Can you work these out from the model? Positions are in its coordinate system, mm. Face numbers are marked on the shaded views. A direction names the side the tool comes from. Round coordinates to 2 decimals unless told otherwise and drop trailing zeros. Write each loop counter-clockwise with the first axis right and the second up, starting at its lowest first coordinate (ties: lowest second). Pieces come first, ordered by that corner, then holes.
Q1. If we section it at D-D (x = -37): Please give me the cut outline in (y, z).
Q2. If we section it at A-A (x = 2.5): Please give me the cut outline in (y, z).
Q3. If we section it at C-C (y = 36.5): Please give me the cut outline in (x, z), plus the area to 3 significant figures.
Q4. I'm going to push flat-ended pins straight in: pin 1 Ø1.5 at (x, z) = (44.5, 13) entering from -Y; pin 2 Ø1.6 at (x, y) = (47, 51) entering from -Z. Where does each tip first touch, or does it pass through?
Q5. If we section it at B-B (z = 42): Please give me the cut outline in (x, y).
Q6. For the marked faces 1, 2 and 3, which set-ups out of +Z, -Z, +X, -X, +Y, -Y let a thin tool reach every point of the face, with its end or its side?
Q7. We'd pull the mould along X, two halves only. Please class the marked faces 4, 5 and 6: +X half, -X half, draft (parallel to the pull), parting line (faces both ways), or undercut.
Q8. Please list where these lines run through material, in increasing order: line 1 along X through (y, z) = (2.05, 0); line 2 along Y through (x, z) = (4.5, 31.5); line 3 along Z through (x, y) = (-2, 38.5).
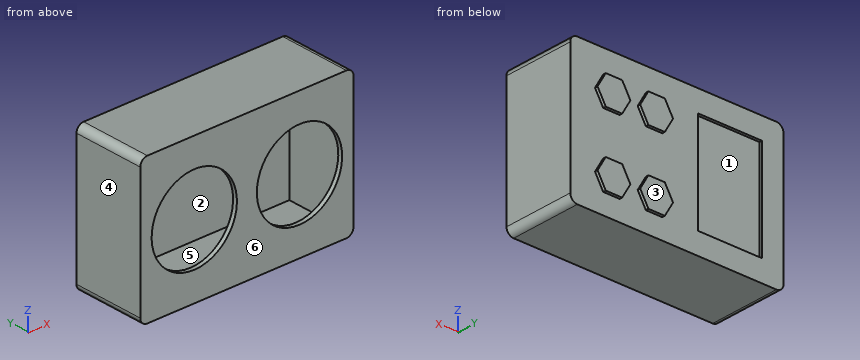
from build123d import *

# Parameters (mm, degrees)
SKETCH1_W           = 150
SKETCH1_H           = 100
BOSS_EXTRUDE1_DEPTH = 50
SHELL1_T            = 3
SKETCH3_R           = 30
CUT_EXTRUDE2_DEPTH  = 5
SKETCH4_W           = 45
SKETCH4_H           = 70
CUT_EXTRUDE3_DEPTH  = 2
BOSS_EXTRUDE2_DEPTH = 2
FILLET1_R           = 5


with BuildPart() as part:
    # Sketch1 → Boss-Extrude1 (new body)
    with BuildSketch(Plane(origin=(0, 0, 0), x_dir=(1, 0, 0), z_dir=(0, 1, 0))):
        Rectangle(SKETCH1_W, SKETCH1_H)
    extrude(amount=BOSS_EXTRUDE1_DEPTH)

    # Shell1 (no face opened: a closed hollow body)
    add(offset(amount=-SHELL1_T, mode=Mode.PRIVATE), mode=Mode.SUBTRACT)

    # Sketch3 → Cut-Extrude2 (cut)
    with BuildSketch(Plane.XZ):
        with Locations(Location((37, 0, 0), (0, 0, 270))):
            Circle(SKETCH3_R)
        with Locations(Location((-37, 0, 0), (0, 0, 270))):
            Circle(SKETCH3_R)
    extrude(amount=-CUT_EXTRUDE2_DEPTH, mode=Mode.SUBTRACT)

    # Sketch4 → Cut-Extrude3 (cut)
    with BuildSketch(Plane(origin=(0, 50, 0), x_dir=(1, 0, 0), z_dir=(0, 1, 0))):
        with Locations((-37.5, 0)):
            Rectangle(SKETCH4_W, SKETCH4_H)
    extrude(amount=-CUT_EXTRUDE3_DEPTH, mode=Mode.SUBTRACT)

    # Sketch5 → Boss-Extrude2 (add)
    with BuildSketch(Plane(origin=(0, 50, 0), x_dir=(1, 0, 0), z_dir=(0, 1, 0))):
        Polygon((57.58863582, -24), (51.815133128, -14), (40.268127744, -14), (34.494625052, -24), (40.268127744, -34), (51.815133128, -34), align=None)
        Polygon((27.58863582, -24), (21.815133128, -14), (10.268127744, -14), (4.494625052, -24), (10.268127744, -34), (21.815133128, -34), align=None)
        Polygon((57.58863582, 26), (51.815133128, 36), (40.268127744, 36), (34.494625052, 26), (40.268127744, 16), (51.815133128, 16), align=None)
        Polygon((27.58863582, 26), (21.815133128, 36), (10.268127744, 36), (4.494625052, 26), (10.268127744, 16), (21.815133128, 16), align=None)
    extrude(amount=BOSS_EXTRUDE2_DEPTH)

    # Fillet1
    fillet1_edges = [part.edges().sort_by_distance(p)[0] for p in [
        (75, 25, 50),
        (-75, 25, 50),
        (-75, 25, -50),
        (75, 25, -50),
    ]]
    fillet(fillet1_edges, radius=FILLET1_R)


solid = part.part
A:
1. outline: (0, -50) - (50, -50) - (50, -35) - (48, -35) - (48, 35) - (50, 35) - (50, 50) - (0, 50) - (0, 30) - (3, 30) - (3, 47) - (47, 47) - (47, -47) - (3, -47) - (3, -30) - (0, -30) - close
2. outline: (0, -50) - (50, -50) - (50, 50) - (0, 50) - close; hole (3, -47) - (47, -47) - (47, 47) - (3, 47) - close
3. outline: (-75, -45) arc R5 ccw to (-70, -50) - (70, -50) arc R5 ccw to (75, -45) - (75, 45) arc R5 ccw to (70, 50) - (-70, 50) arc R5 ccw to (-75, 45) - close; hole (-72, -47) - (72, -47) - (72, 47) - (-72, 47) - close
3. area: 1,440 mm2
4. pin 1: stops at y = 47
4. pin 2: stops at z = -36
5. outline: (-75, 0) - (75, 0) - (75, 50) - (-75, 50) - close; hole (-72, 3) - (72, 3) - (72, 47) - (-72, 47) - close
6. face 1: +Y
6. face 2: none
6. face 3: +Z, -Z, +X, -X, +Y
7. face 4: -X half
7. face 5: undercut
7. face 6: draft
8. line 1: x = -75 to -67, -7 to 7, 67 to 75
8. line 2: y = 0 to 3, 47 to 50
8. line 3: z = -50 to -47, 47 to 50
